```python
from build123d import *

# Parameters (mm, degrees)
BOSS_EXTRUDE1_DEPTH = 2.5
SKETCH3_R           = 2
CUT_EXTRUDE1_DEPTH  = 2.5
CIRPATTERN1_COUNT   = 4


with BuildPart() as part:
    # Sketch1 → Boss-Extrude1 (new body)
    with BuildSketch(Plane(origin=(0, 0, 0), x_dir=(1, 0, 0), z_dir=(0, 1, 0))):
        with BuildLine():
            Line((-13.7, 60), (13.7, 60))
            ThreePointArc((13.7, 60), (33.917107936, 33.917107936), (60, 13.7))
            Line((60, 13.7), (60, -13.7))
            ThreePointArc((60, -13.7), (33.917107936, -33.917107936), (13.7, -60))
            Line((13.7, -60), (-13.7, -60))
            ThreePointArc((-13.7, -60), (-33.917107936, -33.917107936), (-60, -13.7))
            Line((-60, -13.7), (-60, 13.7))
            ThreePointArc((-60, 13.7), (-33.917107936, 33.917107936), (-13.7, 60))
        make_face()
    extrude(amount=BOSS_EXTRUDE1_DEPTH)

    # Sketch3 → Cut-Extrude1 (cut)
    with BuildSketch(Plane(origin=(0, 2.5, 0), x_dir=(1, 0, 0), z_dir=(0, 1, 0))):
        with Locations(Location((-8.259716624, 52.5, 0), (0, 0, 270))):
            Circle(SKETCH3_R)
        with Locations(Location((7.740283376, 52.5, 0), (0, 0, 270))):
            Circle(SKETCH3_R)
    cut_extrude1 = extrude(amount=-CUT_EXTRUDE1_DEPTH, mode=Mode.SUBTRACT)

    # CirPattern1: Cut-Extrude1 ×4 about axis
    cirpattern1_axis = Axis((0, 0, 0), (0, 1, 0))
    for i in range(1, CIRPATTERN1_COUNT):
        add(cut_extrude1.rotate(cirpattern1_axis, i * 360 / CIRPATTERN1_COUNT), mode=Mode.SUBTRACT)


solid = part.part
```
Part model, mm, in its own coordinate system. Round coordinates to 2 decimals unless told otherwise and drop trailing zeros. Loops run counter-clockwise (first coordinate to the right, second up) from the corner with the lowest first, then second, coordinate; pieces in that order, holes last. Notation, with made-up numbers: (31, 46.25) -> (74, 46.25) arc R32 ccw to (74, 85.25) -> close; hole circle Ø3 at (44, -6). An arc over 180 degrees is marked (long way). Use CSV: the item, a comma, the result in double quotes. Start each with the question number.
1) Cut at D-D, the plane x = -31.5. Write the cut outline in (y, z), plus the area to 3 significant figures.
2) Drop a flat-ended pin along its axis: P1, Ø5, axis at x = 8.26, z = 52.5, coming from the -Y side. Give the stop position or say it passes through.
3) Cut at B-B, the plane y = 1.35. Give the number of separate pieces and of enclosed holes in the cut face, plus the area to 3 significant figures.
4) Cut at A-A, the plane z = -52.5. Write the cut outline in (x, y), plus the area to 3 significant figures.
5) Cut at C-C, the plane x = -52.5. Write the cut outline in (y, z).
6) Wall check: L1, parallel to Z at x = 8, y = 1.3; L2, parallel to X at y = 1.9, z = -52.5; L3, parallel to Z at x = -52.5, y = 0.8. Give the ranges that are in metal, low to high. Write a range as [from, to].
Determined:
1,outline,"(0, -36.4) -> (2.5, -36.4) -> (2.5, 36.4) -> (0, 36.4) -> close"
1,area,"182 mm2"
2,P1,"stops at y = 0"
3,separate pieces,"1"
3,enclosed holes,"8"
3,area,"9,290 mm2"
4,outline,"(-18.48, 0) -> (-10.26, 0) -> (-10.26, 2.5) -> (-18.48, 2.5) -> close; (-6.26, 0) -> (5.74, 0) -> (5.74, 2.5) -> (-6.26, 2.5) -> close; (9.74, 0) -> (18.48, 0) -> (18.48, 2.5) -> (9.74, 2.5) -> close"
4,area,"72.4 mm2"
5,outline,"(0, -18.48) -> (2.5, -18.48) -> (2.5, -9.74) -> (0, -9.74) -> close; (0, -5.74) -> (2.5, -5.74) -> (2.5, 6.26) -> (0, 6.26) -> close; (0, 10.26) -> (2.5, 10.26) -> (2.5, 18.48) -> (0, 18.48) -> close"
6,L1,"z = [-60, -54.48], [-50.52, 50.52], [54.48, 60]"
6,L2,"x = [-18.48, -10.26], [-6.26, 5.74], [9.74, 18.48]"
6,L3,"z = [-18.48, -9.74], [-5.74, 6.26], [10.26, 18.48]"
